```python
from build123d import *

# Parameters (mm, degrees)
SKETCH1_W           = 90
SKETCH1_H           = 30
SKETCH1_W_2         = 30
SKETCH1_R           = 5
BOSS_EXTRUDE1_DEPTH = 30
FILLET1_R           = 10


with BuildPart() as part:
    # Sketch1 → Boss-Extrude1 (new body)
    # profile 1 of 3: a face of its own
    with BuildSketch(Plane(origin=(0, 0, 0), x_dir=(1, 0, 0), z_dir=(0, 1, 0))):
        Rectangle(SKETCH1_W, SKETCH1_H)
    # profile 2 of 3: a face of its own
    with BuildSketch(Plane(origin=(0, 0, 0), x_dir=(1, 0, 0), z_dir=(0, 1, 0))):
        with Locations((60, 0)):
            Rectangle(SKETCH1_W_2, SKETCH1_H)
        with Locations(Location((60, 0, 0), (0, 0, 270))):
            Circle(SKETCH1_R, mode=Mode.SUBTRACT)
    # profile 3 of 3: a face of its own
    with BuildSketch(Plane(origin=(0, 0, 0), x_dir=(1, 0, 0), z_dir=(0, 1, 0))):
        with Locations((-60, 0)):
            Rectangle(SKETCH1_W_2, SKETCH1_H)
        with Locations(Location((-60, 0, 0), (0, 0, 270))):
            Circle(SKETCH1_R, mode=Mode.SUBTRACT)
    extrude(amount=BOSS_EXTRUDE1_DEPTH)

    # Fillet1
    fillet1_edges = [part.edges().sort_by_distance(p)[0] for p in [
        (-75, 15, 15),
        (-75, 15, -15),
        (75, 15, -15),
        (75, 15, 15),
    ]]
    fillet(fillet1_edges, radius=FILLET1_R)


solid = part.part
```
Geometry: final body of the model. Coordinates: model frame, mm. Round coordinates to 2 decimals unless told otherwise and drop trailing zeros. Order: outer loops, then holes, each group sorted by start corner. A loop starts at its lowest first (then second) coordinate and runs counter-clockwise, first axis right, second up. Notation, with made-up numbers: (9, 17) -> (35, 17) arc R37 ccw to (35, 56) -> close; hole circle Ø10 at (48, 1). An arc over 180 degrees is marked (long way). Use one line per item in the form item = value.
(1) Section D-D on z = -11. Return loops of the section in (x, y).
Results list:
outline = (-73, 0) -> (73, 0) -> (73, 30) -> (-73, 30) -> close
(2) Section B-B on y = 21.75. Return loops of the section in (x, z), and give its area (3 significant figures).
Results list:
outline = (-75, -5) arc R10 ccw to (-65, -15) -> (65, -15) arc R10 ccw to (75, -5) -> (75, 5) arc R10 ccw to (65, 15) -> (-65, 15) arc R10 ccw to (-75, 5) -> close; hole circle Ø10 at (-60, 0); hole circle Ø10 at (60, 0)
area = 4,260 mm^2
(3) Section A-A on x = -60. Return loops of the section in (y, z), and give its area (3 significant figures).
Results list:
outline = (0, -15) -> (30, -15) -> (30, -5) -> (0, -5) -> close; (0, 5) -> (30, 5) -> (30, 15) -> (0, 15) -> close
area = 600 mm^2
(4) Draft query along Z for faces 1 (the face through (-1, 15, 15)), 2 (the face through (-72.15, 15.21, -11.99)), 3 (the face through (-1, 30, 0)), 4 (the face through (64, 15, 3)). Return one class per face: pulls with the +Z half, pulls with the -Z half, needs draft (parallel to the pull), parting line crosses it, or undercut.
Results list:
face_1 = pulls with the +Z half
face_2 = pulls with the -Z half
face_3 = needs draft
face_4 = undercut
(5) First-contact query: pin 1 Ø6 at (x, z) = (60, 0) entering from -Y; pin 2 Ø1.5 at (y, z) = (16.5, -9.5) entering from +X; pin 3 Ø1.5 at (y, z) = (12.5, 6.5) entering from -X. Flat tips, straight axial feed; report the tip coordinate or a pass-through.
Results list:
pin_1 = through
pin_2 = 74.27
pin_3 = -74.97
(6) Section C-C on z = -3. Return loops of the section in (x, y), and give its area (3 significant figures).
Results list:
outline = (-75, 0) -> (-64, 0) -> (-64, 30) -> (-75, 30) -> close; (-56, 0) -> (56, 0) -> (56, 30) -> (-56, 30) -> close; (64, 0) -> (75, 0) -> (75, 30) -> (64, 30) -> close
area = 4,020 mm^2
(7) Ray query, probe 1 along X at (y, z) = (21, 0); probe 2 along X at (y, z) = (14.75, -2); probe 3 along Z at (x, y) = (58, 21.25). Return the intervals inside material, ascending. Write a range as [from, to].
Results list:
probe_1 = [-75, -65], [-55, 55], [65, 75]
probe_2 = [-75, -64.58], [-55.42, 55.42], [64.58, 75]
probe_3 = [-15, -4.58], [4.58, 15]
